Design review of the part built by this model. Coordinates are the model's own, in mm. Round coordinates to 2 decimals unless told otherwise and drop trailing zeros. Order: outer loops, then holes, each group sorted by start corner. A loop starts at its lowest first (then second) coordinate and runs counter-clockwise, first axis right, second up. Notation, with made-up numbers: M 41,50 L 50,50 A23 cw 50,84 Z; hole C -8,74 d11. An arc over 180 degrees is marked long. Use a Markdown table: item, result. Add a question column.
(1) Take a section at B-B (x = 960.5). Write out the cut boundary in (y, z), then the cut area to 3 significant figures.
(2) For pin 1 (1.5 mm diameter, centred on y = 2871, z = 11, fed in from -X); pin 2 (8 mm diameter, centred on y = 2767.5, z = 15, fed in from +X); pin 3 (3 mm diameter, centred on y = 2575, z = 8.5, fed in from +X), all flat-tipped, find the tip position at first contact; note any pin that passes through.
(3) Take a section at C-C (z = 5). Count the separate pieces of the cut face and the enclosed holes in it, then the cut area to 3 significant figures.
(4) Take a section at D-D (y = 2886.5). Write out the cut boundary in (x, z).
(5) The part is to be moulded in two halves that separate along Y. For faces 1 (the face through (1472, 2818, 0)), 2 (the face through (740.4, 2822.8, 10)), 3 (the face through (1578.767, 3114.832, 10.018)), say which applies: released by +Y, released by -Y, zero draft, split by the parting line, or undercut.
(6) Take a section at A-A (y = 2699). Write out the cut boundary in (x, z), then the cut area to 3 significant figures.
(7) To check wall thickness, follow probe 1 along X at (y, z) = (2937.5, 12.25); probe 2 along X at (y, z) = (2923.5, 13.75); probe 3 along Y at (x, z) = (959.5, 15.5). State the ranges of each line that lie inside material, in increasing order. Write a range as from..to.
```python
from build123d import *

# Parameters (mm, degrees)
BOSS_EXTRUDE1_DEPTH      = 20.32
CUT_EXTRUDE1_START       = -20.32
CUT_EXTRUDE1_OUTLINE_W   = 112.522
CUT_EXTRUDE1_OUTLINE_H   = 10.16
CUT_EXTRUDE1_OUTLINE_W_2 = 112.4712
CUT_EXTRUDE1_DEPTH       = 20.32
SKETCH3_W                = 10.166490401
SKETCH3_H                = 90.17
SKETCH3_W_2              = 29.273269095
SKETCH3_H_2              = 10.16
SKETCH3_W_3              = 28.575
CUT_EXTRUDE2_DEPTH       = 1125.982


# Read off the part's stored shape, not the designer's step: Cut-Extrude1
with BuildPart() as part:
    # Sketch1 → Boss-Extrude1 (new body)
    with BuildSketch(Plane.XY):
        Polygon((1595.466660195, 3031.488204655), (1326.388576611, 3031.488204655), (1359.327618403, 3195.873483514), (1562.527618403, 3195.873483514), align=None)
        with BuildLine():
            Line((894.428066471, 2570.722953846), (2027.427046989, 2570.722953846))
            add(Edge.make_bspline(
                [(2085.030207364, 2608.219614395), (2082.704936523, 2602.979434666), (2079.555914944, 2597.842123597), (2071.701679737, 2588.506915395), (2066.997802899, 2584.31975945), (2056.553975566, 2577.521356648), (2050.823670006, 2574.916388157), (2039.117489861, 2571.518756347), (2033.151956819, 2570.722953846), (2027.427046989, 2570.722953846)],
                knots=[0, 0, 0, 0, 0.25, 0.25, 0.5, 0.5, 0.75, 0.75, 1, 1, 1, 1], degree=3))
            Line((2085.030207364, 2608.219614395), (2275.234550162, 3031.488204655))
            Line((2275.234550162, 3031.488204655), (646.620686644, 3031.488204655))
            Line((646.620686644, 3031.488204655), (836.825029442, 2608.219614395))
            add(Edge.make_bspline(
                [(836.825029442, 2608.219614395), (839.150300283, 2602.979434666), (842.299321863, 2597.842123597), (850.153557069, 2588.506915395), (854.857433907, 2584.31975945), (865.30126124, 2577.521356648), (871.0315668, 2574.916388157), (882.737746945, 2571.518756347), (888.703279987, 2570.722953846), (894.428066471, 2570.722953846)],
                knots=[0, 0, 0, 0, 0.25, 0.25, 0.5, 0.5, 0.75, 0.75, 1, 1, 1, 1], degree=3))
        make_face()
    extrude(amount=BOSS_EXTRUDE1_DEPTH)

    # Cut-Extrude1 outline → Cut-Extrude1 (cut)
    with BuildSketch(Plane.XY.offset(20.32).offset(CUT_EXTRUDE1_START)):
        Polygon((1629.735958734, 2580.882920539), (1629.73595673, 2570.722953846), (1742.25795673, 2570.722953846), (1742.257958734, 2580.882898338), align=None)
        with Locations((1235.85815673, 2575.802953846)):
            Rectangle(CUT_EXTRUDE1_OUTLINE_W, CUT_EXTRUDE1_OUTLINE_H)
        with Locations((1460.92755673, 2575.802953846)):
            Rectangle(CUT_EXTRUDE1_OUTLINE_W_2, CUT_EXTRUDE1_OUTLINE_H)
    extrude(amount=CUT_EXTRUDE1_DEPTH, mode=Mode.SUBTRACT)

    # Sketch3 → Cut-Extrude2 (cut)
    with BuildSketch(Plane(origin=(0, 0, 0), x_dir=(-1, 0, 0), z_dir=(0, 0, -1))):
        with Locations((-1174.33046881, 2716.137953846)):
            Rectangle(SKETCH3_W, SKETCH3_H)
        with Locations((-1174.33046881, 2896.477953846)):
            Rectangle(SKETCH3_W, SKETCH3_H)
        with Locations((-1183.883858158, 3026.408204655)):
            Rectangle(SKETCH3_W_2, SKETCH3_H_2)
        with Locations((-1738.320389849, 3026.408204655)):
            Rectangle(SKETCH3_W_3, SKETCH3_H_2)
        with Locations((-1747.524644649, 2896.477953846)):
            Rectangle(SKETCH3_W, SKETCH3_H)
        with Locations((-1747.524644649, 2716.137953846)):
            Rectangle(SKETCH3_W, SKETCH3_H)
        Polygon((-1826.076531052, 3021.328204655), (-1826.099732345, 3031.488204655), (-1899.001104211, 3031.488204655), (-1899.001104211, 3021.328204655), align=None)
        Polygon((-2045.548278228, 3031.488204655), (-2045.548278228, 3021.328204655), (-1971.92567737, 3021.328204655), (-1971.948878664, 3031.488204655), align=None)
    extrude(amount=-CUT_EXTRUDE2_DEPTH, mode=Mode.SUBTRACT)


solid = part.part
```
Verdict:
| question | item | result |
|---|---|---|
| 1 | outline | M 2570.72,0 L 3031.49,0 L 3031.49,20.32 L 2570.72,20.32 Z |
| 1 | area | 9,360 mm^2 |
| 2 | pin 1 | stops at x = 718.4 |
| 2 | pin 2 | stops at x = 2158.4 |
| 2 | pin 3 | stops at x = 2053.76 |
| 3 | separate pieces | 1 |
| 3 | enclosed holes | 4 |
| 3 | area | 684,000 mm^2 |
| 4 | outline | M 711.77,0 L 1169.25,0 L 1169.25,20.32 L 711.77,20.32 Z; M 1179.41,0 L 1742.44,0 L 1742.44,20.32 L 1179.41,20.32 Z; M 1752.61,0 L 2210.08,0 L 2210.08,20.32 L 1752.61,20.32 Z |
| 5 | face 1 | zero draft |
| 5 | face 2 | released by -Y |
| 5 | face 3 | released by +Y |
| 6 | outline | M 796.03,0 L 1169.25,0 L 1169.25,20.32 L 796.03,20.32 Z; M 1179.41,0 L 1742.44,0 L 1742.44,20.32 L 1179.41,20.32 Z; M 1752.61,0 L 2125.82,0 L 2125.82,20.32 L 1752.61,20.32 Z |
| 6 | area | 26,600 mm^2 |
| 7 | probe 1 | x = 688.86..1169.25, 1179.41..1742.44, 1752.61..2233 |
| 7 | probe 2 | x = 695.15..1169.25, 1179.41..1742.44, 1752.61..2226.71 |
| 7 | probe 3 | y = 2570.72..3031.49 |
